Here's how the part is built. I have some questions about the finished solid (model axes, mm). A direction names the side the tool comes from. Round coordinates to 2 decimals unless told otherwise and drop trailing zeros. Loops run counter-clockwise (first coordinate to the right, second up) from the corner with the lowest first, then second, coordinate; pieces in that order, holes last. Notation, with made-up numbers: M -36,24 L -4,24 A32 cw -4,57 Z; hole C 39,-16.5 d6. An arc over 180 degrees is marked long. Answer as a JSON object with one key per item and string values.
from build123d import *

# Parameters (mm, degrees)
BOSS_EXTRUDE2_DEPTH     = 10
CUT_EXTRUDE1_DEPTH      = 67.219332525
CUT_EXTRUDE2_DEPTH      = 2
M3_TAPPED_HOLE1_D       = 2.5
M3_TAPPED_HOLE1_DEPTH   = 9
SKETCH9_R               = 2.5
CUT_EXTRUDE3_DEPTH      = 44.185645763
SKETCH10_R              = 4
CUT_EXTRUDE4_DEPTH      = 53.191953403
CHAMFER1_SIZE           = 1
CUT_EXTRUDE5_REACH      = 54.192
CUT_EXTRUDE5_END_RADIUS = 7
SKETCH13_R              = 1.6
M4_TAPPED_HOLE1_REACH   = 68.219
M4_TAPPED_HOLE1_BORE_R  = 1.65
CUT_EXTRUDE6_REACH      = 68.219
CUT_EXTRUDE6_END_RADIUS = 2.5
SKETCH19_R              = 1.25


# Read off the part's stored shape, not the designer's step: Hole1
with BuildPart() as part:
    # Sketch4 → Boss-Extrude2 (new, symmetric)
    with BuildSketch(Plane.XY):
        Polygon((0, 0), (-19, 0), (-19, 32), (9, 32), (21, -6), (21, -30), (0, -30), align=None)
    extrude(amount=BOSS_EXTRUDE2_DEPTH, both=True)

    # Sketch6 → Cut-Extrude1 (cut, through all)
    with BuildSketch(Plane(origin=(0, 32, 0), x_dir=(1, 0, 0), z_dir=(0, 1, 0))):
        with BuildLine():
            ThreePointArc((-2.291796068, 2), (-10.010587075, 6.926666858), (-16, 0))
            Line((-16, 0), (-2, 0))
            ThreePointArc((-2, 0), (-2.073333142, 1.010587075), (-2.291796068, 2))
        make_face()
        with BuildLine():
            Line((-2, 0), (-16, 0))
            ThreePointArc((-16, 0), (-10.010587075, -6.926666858), (-2.291796068, -2))
            ThreePointArc((-2.291796068, -2), (-2.073333142, -1.010587075), (-2, 0))
        make_face()
    extrude(amount=-CUT_EXTRUDE1_DEPTH, mode=Mode.SUBTRACT)

    # Sketch6<3> → Cut-Extrude2 (cut)
    with BuildSketch(Plane(origin=(0, 32, 0), x_dir=(1, 0, 0), z_dir=(0, 1, 0))):
        with BuildLine():
            ThreePointArc((5, 2), (3.585786438, 1.414213562), (3, 0))
            Line((3, 0), (7, 0))
            ThreePointArc((7, 0), (6.414213562, 1.414213562), (5, 2))
        make_face()
        with BuildLine():
            Line((7, 0), (3, 0))
            ThreePointArc((3, 0), (3.585786438, -1.414213562), (5, -2))
            ThreePointArc((5, -2), (6.414213562, -1.414213562), (7, 0))
        make_face()
        with BuildLine():
            ThreePointArc((-2.291796068, 2), (-2.073333142, 1.010587075), (-2, 0))
            Line((-2, 0), (3, 0))
            ThreePointArc((3, 0), (3.585786438, 1.414213562), (5, 2))
            Line((5, 2), (-2.291796068, 2))
        make_face()
        with BuildLine():
            Line((3, 0), (-2, 0))
            ThreePointArc((-2, 0), (-2.073333142, -1.010587075), (-2.291796068, -2))
            Line((-2.291796068, -2), (5, -2))
            ThreePointArc((5, -2), (3.585786438, -1.414213562), (3, 0))
        make_face()
    extrude(amount=-CUT_EXTRUDE2_DEPTH, mode=Mode.SUBTRACT)

    # M3 Tapped Hole1
    with Locations(Plane(origin=(0, 32, 0), x_dir=(1, 0, 0), z_dir=(0, 1, 0))):
        with Locations((-16, 7), (-16, -7), (5, -7), (5, 7)):
            Hole(M3_TAPPED_HOLE1_D / 2, depth=M3_TAPPED_HOLE1_DEPTH)

    # Sketch9 → Cut-Extrude3 (cut, through all)
    with BuildSketch(Plane.XY.offset(10)):
        with Locations((13, -10)):
            Circle(SKETCH9_R)
    extrude(amount=-CUT_EXTRUDE3_DEPTH, mode=Mode.SUBTRACT)

    # Sketch10 → Cut-Extrude4 (cut, through all)
    with BuildSketch(Plane(origin=(21, 0, 0), x_dir=(0, 0, -1), z_dir=(1, 0, 0))):
        with Locations(Location((0, -20, 0), (0, 0, 90))):
            Circle(SKETCH10_R)
    extrude(amount=-CUT_EXTRUDE4_DEPTH, mode=Mode.SUBTRACT)

    # Chamfer1
    chamfer1_edges = [part.edges().sort_by_distance(p)[0] for p in [
        (21, -24, 0),
    ]]
    chamfer(chamfer1_edges, length=CHAMFER1_SIZE)

    # Hole1 outline → Hole1 (revolve, cut)
    with BuildSketch(Plane(origin=(5, 0, 0), x_dir=(1, 0, 0), z_dir=(0, 0, 1))):
        Polygon((1.25, 0), (2, 0), (2, 32), (0, 32), (0, -16.200355886), (1.25, -16.200355886), align=None)
    revolve(axis=Axis((5, 0, 0), (0, 1, 0)), mode=Mode.SUBTRACT)

    # Cut-Extrude5: up to this cylinder (the profile starts outside it)
    cut_extrude5_end = Plane(origin=(-9, 15, 0), z_dir=(0, 1, 0)) * Cylinder(CUT_EXTRUDE5_END_RADIUS, 123.384, mode=Mode.PRIVATE)
    # Sketch13 → Cut-Extrude5 (cut, up to the surface)
    with BuildSketch(Plane.ZY.offset(19), mode=Mode.PRIVATE) as cut_extrude5_sk1:
        with Locations((-3, 15)):
            Circle(SKETCH13_R)
    cut_extrude5_tool1 = extrude(cut_extrude5_sk1.sketch, amount=-CUT_EXTRUDE5_REACH, mode=Mode.PRIVATE) - cut_extrude5_end
    add(cut_extrude5_tool1.solids().sort_by_distance((-19, 15, -3))[0], mode=Mode.SUBTRACT)
    # Sketch13 → Cut-Extrude5 (cut, up to the surface)
    with BuildSketch(Plane.ZY.offset(19), mode=Mode.PRIVATE) as cut_extrude5_sk2:
        with Locations((3, 15)):
            Circle(SKETCH13_R)
    cut_extrude5_tool2 = extrude(cut_extrude5_sk2.sketch, amount=-CUT_EXTRUDE5_REACH, mode=Mode.PRIVATE) - cut_extrude5_end
    add(cut_extrude5_tool2.solids().sort_by_distance((-19, 15, 3))[0], mode=Mode.SUBTRACT)

    # M4 Tapped Hole1 bore → M4 Tapped Hole1 (cut, up to next)
    with BuildSketch(Plane(origin=(0, -30, 0), x_dir=(-1, 0, 0), z_dir=(0, -1, 0)), mode=Mode.PRIVATE) as m4_tapped_hole1_sk1:
        with Locations((-13, 0)):
            Circle(M4_TAPPED_HOLE1_BORE_R)
    m4_tapped_hole1_tool1 = extrude(m4_tapped_hole1_sk1.sketch, amount=-M4_TAPPED_HOLE1_REACH, mode=Mode.PRIVATE) & part.part
    # M4 Tapped Hole1 bore → M4 Tapped Hole1 (cut, up to next)
    with BuildSketch(Plane(origin=(0, -30, 0), x_dir=(-1, 0, 0), z_dir=(0, -1, 0)), mode=Mode.PRIVATE) as m4_tapped_hole1_sk2:
        with Locations((-5, 0)):
            Circle(M4_TAPPED_HOLE1_BORE_R)
    m4_tapped_hole1_tool2 = extrude(m4_tapped_hole1_sk2.sketch, amount=-M4_TAPPED_HOLE1_REACH, mode=Mode.PRIVATE) & part.part
    add(m4_tapped_hole1_tool1.solids().sort_by_distance((13, -30, 0))[0], mode=Mode.SUBTRACT)
    add(m4_tapped_hole1_tool2.solids().sort_by_distance((5, -30, 0))[0], mode=Mode.SUBTRACT)

    # Cut-Extrude6: up to this cylinder (the profile starts outside it)
    cut_extrude6_end = Plane(origin=(13, -10, 0), z_dir=(0, 0, 1)) * Cylinder(CUT_EXTRUDE6_END_RADIUS, 142.438, mode=Mode.PRIVATE)
    # Sketch19 → Cut-Extrude6 (cut, up to the surface)
    with BuildSketch(Plane.XZ.offset(30), mode=Mode.PRIVATE) as cut_extrude6_sk1:
        with Locations((13, 0)):
            Circle(SKETCH19_R)
    cut_extrude6_tool1 = extrude(cut_extrude6_sk1.sketch, amount=-CUT_EXTRUDE6_REACH, mode=Mode.PRIVATE) - cut_extrude6_end
    add(cut_extrude6_tool1.solids().sort_by_distance((13, -30, 0))[0], mode=Mode.SUBTRACT)


solid = part.part
Item 1: If I drill on L1, parallel to X at y = -25.25, z = 0; L2, parallel to Z at x = -17, y = 15; L3, parallel to X at y = -9.75, z = 0, over which ranges is the centre line in solid material (lowest first)? Write a range as from..to.
Solution:
{"L1": "x = 0..3.35, 6.65..11.35, 14.65..21", "L2": "z = -10..-4.6, -1.4..1.4, 4.6..10", "L3": "x = 0..3.75, 6.25..10.51, 15.49..21"}
Item 2: I want a section at A-A on y = 15. List the corners of the cut face in (x, z) for me.
Solution:
{"outline": "M -19,-10 L 14.37,-10 L 14.37,10 L -19,10 L -19,4.6 L -14.28,4.6 A7 cw long -14.28,-4.6 L -19,-4.6 Z; M -19,-1.4 L -15.86,-1.4 A7 cw -15.86,1.4 L -19,1.4 Z; hole C 5,0 d4"}
Item 3: For faces 1 (the face through (6.65, -26.87, -0.07)), 2 (the face through (-16, 23, 7)), 3 (the face through (1, 1, 10)), 4 (the face through (0, -15, 0)), which set-ups out of +Z, -Z, +X, -X, +Y, -Y let a thin tool reach every point of the face, with its end or its side?
Solution:
{"face 1": "-Y", "face 2": "+Y", "face 3": "+Z, +X, -X, +Y, -Y", "face 4": "+Z, -Z, -X, -Y"}
Item 4: For P1, Ø1.2, axis at x = 5.5, z = -7, coming from the +Y side; P2, Ø10, axis at x = -12, z = 5, coming from the -Y side; P3, Ø6, axis at y = -22.5, z = -1.5, coming from the -X side, each with a flat end and sliding along its axis, tell me the tip position at first contact or that it passes through.
Solution:
{"P1": "stops at y = 23", "P2": "stops at y = 0", "P3": "stops at x = 0"}
Item 5: We'd pull the mould along Z, two halves only. Please class faces 5 (the face through (-17.196, 15.481, 4.526)), 6 (the face through (1, 1, -10)), 7 (the face through (12.67, -7.52, 0.14)): +Z half, -Z half, draft (parallel to the pull), parting line (faces both ways), or undercut.
Solution:
{"face 5": "undercut", "face 6": "-Z half", "face 7": "draft"}
Item 6: I want a section at D-D on y = 4.5. List the corners of the cut face in (x, z) for me, plus the area to 3 significant figures.
Solution:
{"outline": "M -19,-10 L 17.68,-10 L 17.68,10 L -19,10 Z; hole C -9,0 d14; hole C 5,0 d4", "area": "567 mm2"}
Item 7: I want a section at C-C on x = 8. List the corners of the cut face in (y, z) for me.
Solution:
{"outline": "M -30,-10 L 32,-10 L 32,10 L -30,10 Z; hole C -20,0 d8"}
Item 8: I want a section at B-B on x = -8. List the corners of the cut face in (y, z) for me, plus the area to 3 significant figures.
Solution:
{"outline": "M 0,-10 L 32,-10 L 32,-6.93 L 0,-6.93 Z; M 0,6.93 L 32,6.93 L 32,10 L 0,10 Z", "area": "197 mm2"}
